Input: part model. Units: mm. Frame: model coordinates. A direction names the side the tool comes from. Give positions to 0.01 mm unless a question says otherwise; leave off trailing zeros. Write each loop counter-clockwise with the first axis right and the second up, starting at its lowest first coordinate (ties: lowest second). Pieces come first, ordered by that corner, then holes. Notation, with made-up numbers: (80, 70.5) -> (104, 70.5) arc R13 cw to (104, 82.5) -> close; hole circle Ø5 at (-25, 89). An arc over 180 degrees is marked (long way). Return JSON: item names as keys, results as strings. Group by question number.
Item 1: Line query: line 1 (X direction, y = -2.75, z = 6.5); line 2 (Z direction, x = -21.75, y = 1.75); line 3 (Z direction, x = -15.5, y = -2.5). Output: solid intervals per line, ascending. Write a range as [from, to].
Item 2: Mould query, pull axis X, two halves, no side actions, for faces 5 (the face through (-13.19, 2.03, 12.21)), 6 (the face through (-11.159, 0, 10)), 7 (the face through (-21, 0, 12)). Classes: released by +X, released by -X, zero draft, split by the parting line, or undercut.
Item 3: Set-up query: faces 1 (the face through (-26.557, 0.087, 13.972)), 2 (the face through (-15.159, 3, 12)), 3 (the face through (-25, 0, 16)), 4 (the face through (-26.557, 0.087, 6.028)). Return all of +Z, -Z, +X, -X, +Y, -Y with unobstructed straight access to the full face (end or side cutting, diameter ignored); none if empty.
Item 4: Pin query (flat end, axial travel): P1, Ø0.6, axis at y = 2, z = 12.5, coming from the -X side; P2, Ø1.5, axis at y = 3, z = 5.5, coming from the -X side; P3, Ø5, axis at x = -14.5, z = 8.5, coming from the +Y side; P4, Ø1.6, axis at y = -1.5, z = 6.5, coming from the -X side. Return the tip coordinate at first contact, or that it passes through.
Item 5: Section B-B, the plane z = 10. Return loops of the section in (x, y), then the cut area to 3 significant figures.
Item 6: Section C-C, the plane x = -24. Return loops of the section in (y, z).
Item 7: Section D-D, the plane z = 7.5. Return loops of the section in (x, y).
Item 8: Section A-A, the plane z = 13.5. Return loops of the section in (x, y), then the cut area to 3 significant figures.
from build123d import *

# Parameters (mm, degrees)
BOSS_EXTRUDE1_DEPTH = 20
SKETCH2_R           = 10
BOSS_EXTRUDE2_DEPTH = 20
SKETCH3_W           = 40.597946668
SKETCH3_H           = 40
BOSS_EXTRUDE3_DEPTH = 5
SKETCH4_R           = 15
BOSS_EXTRUDE4_DEPTH = 20
FILLET1_R           = 1
L_EK2_SCALE         = 0.2


with BuildPart() as part:
    # Sketch1 → Boss-Extrude1 (new body)
    with BuildSketch(Plane.XY):
        with BuildLine():
            Line((-42, 20), (0, 20))
            Line((0, 20), (0, -20))
            Line((0, -20), (-42, -20))
            ThreePointArc((-42, -20), (-62, 0), (-42, 20))
        make_face()
    extrude(amount=BOSS_EXTRUDE1_DEPTH)

    # Sketch2 → Boss-Extrude2 (add)
    with BuildSketch(Plane.XY.offset(20)):
        with Locations((-42, 0)):
            Circle(SKETCH2_R)
    boss_extrude2 = extrude(amount=BOSS_EXTRUDE2_DEPTH)

    # Mirror1: Boss-Extrude2 across plane
    add(boss_extrude2.mirror(Plane.XY.offset(10)))

    # Sketch3 → Boss-Extrude3 (add)
    with BuildSketch(Plane(origin=(0, 0, 0), x_dir=(0, 0, -1), z_dir=(1, 0, 0))):
        with Locations((-10, 0)):
            Rectangle(SKETCH3_W, SKETCH3_H)
    extrude(amount=BOSS_EXTRUDE3_DEPTH)

    # Sketch4 → Boss-Extrude4 (add)
    with BuildSketch(Plane(origin=(5, 0, 0), x_dir=(0, 0, -1), z_dir=(1, 0, 0))):
        with Locations((-10, 0)):
            Circle(SKETCH4_R)
    extrude(amount=BOSS_EXTRUDE4_DEPTH)

    # Fillet1
    fillet1_edges = [part.edges().sort_by_distance(p)[0] for p in [
        (-21, 20, 20),
        (0, 0, -10.298973334),
        (0, 20, -5.149486667),
        (0, 20, 25.149486667),
        (2.5, 20, -10.298973334),
        (0, 0, 30.298973334),
        (2.5, 20, 30.298973334),
        (5, 0, -10.298973334),
        (5, 20, 10),
        (5, 0, 30.298973334),
        (5, -20, 10),
        (-62, 0, 20),
        (-21, 20, 0),
        (-21, -20, 0),
        (-62, 0, 0),
        (-21, -20, 20),
    ]]
    fillet(fillet1_edges, radius=FILLET1_R)


with BuildPart() as part_1:
    # Ölçek2: scaled about (-20.19862857, -0.001535567, 10)
    add(part.part.scale(L_EK2_SCALE).moved(Location((-16.158902856, -0.001228454, 8))))


solid = part_1.part
Answer below:
{
 "1": {"line 1": "x = [-16.16, -15.16]", "line 2": "z = [8, 12]", "line 3": "z = [5.94, 14.06]"},
 "2": {"face 5": "zero draft", "face 6": "released by +X", "face 7": "undercut"},
 "3": {"face 1": "+Z", "face 2": "+X", "face 3": "+Z, +X, -X, +Y, -Y", "face 4": "-Z"},
 "4": {"P1": "stops at x = -25.61", "P2": "stops at x = -16.16", "P3": "stops at y = 4", "P4": "stops at x = -26.43"},
 "5": {"outline": "(-24.56, -4) -> (-15.36, -4) arc R0.2 ccw to (-15.16, -3.8) -> (-15.16, -3) -> (-11.16, -3) -> (-11.16, 3) -> (-15.16, 3) -> (-15.16, 3.8) arc R0.2 ccw to (-15.36, 4) -> (-24.56, 4) arc R4 ccw to start", "area": "124 mm2"},
 "6": {"outline": "(-4, 8.2) arc R0.2 ccw to (-3.8, 8) -> (-1.92, 8) -> (-1.92, 4) -> (1.92, 4) -> (1.92, 8) -> (3.8, 8) arc R0.2 ccw to (4, 8.2) -> (4, 11.8) arc R0.2 ccw to (3.8, 12) -> (1.92, 12) -> (1.92, 16) -> (-1.92, 16) -> (-1.92, 12) -> (-3.8, 12) arc R0.2 ccw to (-4, 11.8) -> close"},
 "7": {"outline": "circle Ø4 at (-24.56, 0); (-16.16, -4) -> (-15.36, -4) arc R0.2 ccw to (-15.16, -3.8) -> (-15.16, -1.66) -> (-11.16, -1.66) -> (-11.16, 1.66) -> (-15.16, 1.66) -> (-15.16, 3.8) arc R0.2 ccw to (-15.36, 4) -> (-15.96, 4) arc R0.2 ccw to (-16.16, 3.8) -> close"},
 "8": {"outline": "circle Ø4 at (-24.56, 0); (-16.16, -4) -> (-15.36, -4) arc R0.2 ccw to (-15.16, -3.8) -> (-15.16, 3.8) arc R0.2 ccw to (-15.36, 4) -> (-15.96, 4) arc R0.2 ccw to (-16.16, 3.8) -> close", "area": "20.5 mm2"}
}
